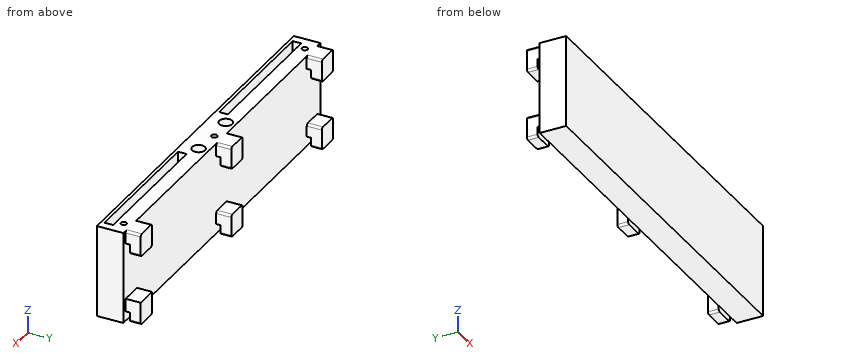
from build123d import *

# Parameters (mm, degrees)
F0_W      = 174
F0_H      = 12.3
F1_DEPTH  = 42.8
F2_W      = 10
F2_H      = 10.5
F3_DEPTH  = 7
F4_W      = 2
F4_H      = 4.5
F5_DEPTH  = 172.001
F6_W      = 65
F6_H      = 4
F6_R      = 1.35
F7_DEPTH  = 13
F8_R      = 1
F9_R      = 3
F10_DEPTH = 38


with BuildPart() as f1:
    # F0 (on Top) → F1 (new body)
    with BuildSketch(Plane.XY):
        with Locations((0, -6.15)):
            Rectangle(F0_W, F0_H)
    extrude(amount=F1_DEPTH)

    # F2 (on face) → F3 (join)
    with BuildSketch(Plane(origin=(0, 0, 0), x_dir=(-1, 0, 0), z_dir=(0, 1, 0))):
        with Locations((80, 37.55)):
            Rectangle(F2_W, F2_H)
        with Locations((0, 37.55)):
            Rectangle(F2_W, F2_H)
        with Locations((-80, 37.55)):
            Rectangle(F2_W, F2_H)
        with Locations((80, 5.25)):
            Rectangle(F2_W, F2_H)
        with Locations((0, 5.25)):
            Rectangle(F2_W, F2_H)
        with Locations((-80, 5.25)):
            Rectangle(F2_W, F2_H)
    extrude(amount=F3_DEPTH)

    # F4 (on face) → F5 (cut, through all)
    with BuildSketch(Plane.YZ.offset(85)):
        with Locations((1, 34.55)):
            Rectangle(F4_W, F4_H)
        with Locations((1, 2.25)):
            Rectangle(F4_W, F4_H)
    extrude(amount=-F5_DEPTH, mode=Mode.SUBTRACT)

    # F6 (on face) → F7 (cut)
    with BuildSketch(Plane.XY.offset(42.8)):
        with Locations((-50.65, -8.8)):
            Rectangle(F6_W, F6_H)
        with Locations((50.65, -8.8)):
            Rectangle(F6_W, F6_H)
        with Locations((-80, -3.5)):
            Circle(F6_R)
        with Locations((0, -3.5)):
            Circle(F6_R)
        with Locations((80, -3.5)):
            Circle(F6_R)
    extrude(amount=-F7_DEPTH, mode=Mode.SUBTRACT)

    # F8
    f8_edges = [f1.edges().sort_by_distance(p)[0] for p in [
        (-5, 3.5, 42.8),
        (5, 3.5, 42.8),
        (-75, 3.5, 42.8),
        (-85, 3.5, 42.8),
        (75, 3.5, 42.8),
        (85, 3.5, 42.8),
        (5, 3.5, 10.5),
        (-5, 3.5, 10.5),
        (-75, 3.5, 10.5),
        (-85, 3.5, 10.5),
        (85, 4.5, 32.3),
        (85, 4.5, 0),
        (75, 4.5, 0),
        (5, 4.5, 32.3),
        (5, 4.5, 0),
        (-5, 4.5, 0),
        (-75, 4.5, 32.3),
        (-75, 4.5, 0),
        (-85, 4.5, 0),
        (-85, 4.5, 32.3),
        (-5, 4.5, 32.3),
        (75, 4.5, 32.3),
    ]]
    fillet(f8_edges, radius=F8_R)

    # F9 (on face) → F10 (cut)
    with BuildSketch(Plane.XY.offset(42.8)):
        with Locations((12, -4.5)):
            Circle(F9_R)
        with Locations((-12, -4.5)):
            Circle(F9_R)
    extrude(amount=-F10_DEPTH, mode=Mode.SUBTRACT)


solid = f1.part
Source: CAD feature listing. Evaluate the final solid. Frame: model axes, mm. Round coordinates to 2 decimals unless told otherwise and drop trailing zeros. Loops run counter-clockwise (first coordinate to the right, second up) from the corner with the lowest first, then second, coordinate; pieces in that order, holes last.
Q1. Section B-B, the plane z = 26.5. Return loops of the section in (x, y).
Q2. First-contact query: P1, Ø3.5, axis at y = 2.5, z = 4, coming from the +X side; P2, Ø5.5, axis at y = 4, z = 36, coming from the -X side; P3, Ø2.5, axis at x = -80, y = -3.5, coming from the +Z side. Flat tips, straight axial feed; report the tip coordinate or a pass-through.
Q3. Ray query, line 1 (X direction, y = 5.5, z = 5.5); line 2 (Y direction, x = 0, z = 33); line 3 (X direction, y = -10.5, z = 37.5). Return the intervals inside material, ascending.
Q4. Section A-A, the plane x = -34.5. Return loops of the section in (y, z).
Q5. Section C-C, the plane x = 12. Return loops of the section in (y, z).
Solutions:
1. outline: (-87, -12.3) - (87, -12.3) - (87, 0) - (-87, 0) - close; hole circle Ø6 at (-12, -4.5); hole circle Ø6 at (12, -4.5)
2. P1: stops at x = 85
2. P2: stops at x = -85
2. P3: stops at z = 29.8
3. line 1: x = -85 to -75, -5 to 5, 75 to 85
3. line 2: y = -12.3 to -4.85, -2.15 to 0, 2 to 7
3. line 3: x = -87 to -83.15, -18.15 to 18.15, 83.15 to 87
4. outline: (-12.3, 0) - (0, 0) - (0, 42.8) - (-6.8, 42.8) - (-6.8, 29.8) - (-10.8, 29.8) - (-10.8, 42.8) - (-12.3, 42.8) - close
5. outline: (-12.3, 0) - (0, 0) - (0, 42.8) - (-1.5, 42.8) - (-1.5, 4.8) - (-7.5, 4.8) - (-7.5, 42.8) - (-12.3, 42.8) - close
